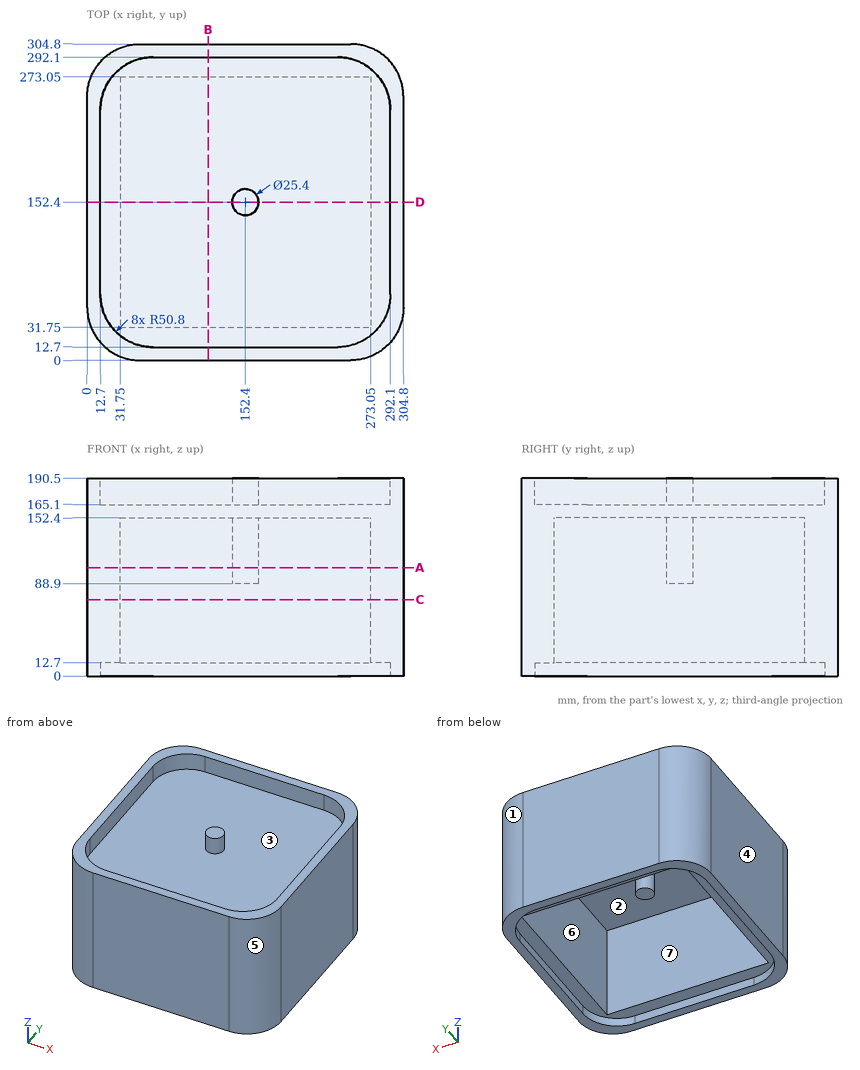
Job drawing, mm, ordinate dimensions from the low corner. One solid piece. A direction names the side the tool comes from. Round coordinates to 2 decimals unless told otherwise and drop trailing zeros. Loops run counter-clockwise (first coordinate to the right, second up) from the corner with the lowest first, then second, coordinate; pieces in that order, holes last.
Item 1: Cut at A-A, the plane z = 104.5. Give the cut face in (x, y), then the cut area to 3 significant figures.
Item 2: Cut at C-C, the plane z = 73.5. Give the cut face in (x, y).
Item 3: Mould opens along X. For the marked faces 4, 5, 6 and 7 say: +X half, -X half, draft (parallel to the pull), parting line (faces both ways), or undercut.
Item 4: Drill centre lines: line 1 (X direction, y = 189.5, z = 103); line 2 (Y direction, x = 155.5, z = 128.5). Where is each one in solid material? Low to high.
Item 5: Cut at D-D, the plane y = 152.4. Give the cut face in (x, z), then the cut area to 3 significant figures.
Item 6: Drop flat-ended pins along their axis: P1, Ø10, axis at x = 185, y = 112.5, coming from the -Z side; P2, Ø5, axis at y = 43, z = 54.5, coming from the -X side. Give the stop position or say it passes through.
Item 7: 3-axis set-ups, long thin cutter, end or side, ignore diameter. For the marked faces 1, 2 and 3: which of +Z, -Z, +X, -X, +Y, -Y reach the whole face in a straight line?
Item 8: Cut at B-B, the plane x = 116.5. Give the cut face in (y, z).
A:
1. outline: (0, 50.8) arc R50.8 ccw to (50.8, 0) - (254, 0) arc R50.8 ccw to (304.8, 50.8) - (304.8, 254) arc R50.8 ccw to (254, 304.8) - (50.8, 304.8) arc R50.8 ccw to (0, 254) - close; circle Ø25.4 at (152.4, 152.4); hole (31.75, 31.75) - (273.05, 31.75) - (273.05, 273.05) - (31.75, 273.05) - close
1. area: 33,000 mm2
2. outline: (0, 50.8) arc R50.8 ccw to (50.8, 0) - (254, 0) arc R50.8 ccw to (304.8, 50.8) - (304.8, 254) arc R50.8 ccw to (254, 304.8) - (50.8, 304.8) arc R50.8 ccw to (0, 254) - close; hole (31.75, 31.75) - (273.05, 31.75) - (273.05, 273.05) - (31.75, 273.05) - close
3. face 4: -X half
3. face 5: +X half
3. face 6: undercut
3. face 7: undercut
4. line 1: x = 0 to 31.75, 273.05 to 304.8
4. line 2: y = 0 to 31.75, 140.08 to 164.72, 273.05 to 304.8
5. outline: (0, 0) - (12.7, 0) - (12.7, 12.7) - (31.75, 12.7) - (31.75, 152.4) - (139.7, 152.4) - (139.7, 88.9) - (165.1, 88.9) - (165.1, 152.4) - (273.05, 152.4) - (273.05, 12.7) - (292.1, 12.7) - (292.1, 0) - (304.8, 0) - (304.8, 190.5) - (292.1, 190.5) - (292.1, 165.1) - (165.1, 165.1) - (165.1, 190.5) - (139.7, 190.5) - (139.7, 165.1) - (12.7, 165.1) - (12.7, 190.5) - (0, 190.5) - close
5. area: 16,000 mm2
6. P1: stops at z = 152.4
6. P2: stops at x = 0.28
7. face 1: +Z, -Z, +X, +Y
7. face 2: -Z
7. face 3: +Z
8. outline: (0, 0) - (12.7, 0) - (12.7, 12.7) - (31.75, 12.7) - (31.75, 152.4) - (273.05, 152.4) - (273.05, 12.7) - (292.1, 12.7) - (292.1, 0) - (304.8, 0) - (304.8, 190.5) - (292.1, 190.5) - (292.1, 165.1) - (12.7, 165.1) - (12.7, 190.5) - (0, 190.5) - close
